Build history of the part. All positions in model axes, mm. A direction names the side the tool comes from. Give positions to 0.01 mm unless a question says otherwise; leave off trailing zeros. Order: outer loops, then holes, each group sorted by start corner. A loop starts at its lowest first (then second) coordinate and runs counter-clockwise, first axis right, second up. Notation, with made-up numbers: (87, -6) -> (106, -6) arc R34 ccw to (106, 29) -> close; hole circle Ø7 at (22, 76.25). An arc over 180 degrees is marked (long way). Use a Markdown table: item, result. Add a question column.
Autodesk Inventor part; units mm, degrees
ref_plane "YZ Plane" through (0, 0, 0) normal (1, 0, 0) x (0, 1, 0)
ref_plane "XZ Plane" through (0, 0, 0) normal (0, 1, 0) x (-1, 0, 0)
ref_plane "XY Plane" through (0, 0, 0) normal (0, 0, 1) x (1, 0, 0)
sketch "Sketch1" plane through (0, 0, 0) normal (0, 0, 1) x (1, 0, 0)
  line L0 (-750, 0) -> (750, 0) construction
  line L1 (750, 0) -> (750, -2700) construction
  line L2 (750, -2700) -> (-750, -2700) construction
  line L3 (-750, -2700) -> (-750, 0) construction
  line L4 (800, 50) -> (-800, 50) construction
  line L5 (-800, 50) -> (-800, -2750) construction
  line L6 (-800, -2750) -> (800, -2750) construction
  line L7 (800, -2750) -> (800, 50) construction
  line L8 (-850, 100) -> (850, 100) construction
  line L9 (850, 100) -> (850, -2800) construction
  line L10 (850, -2800) -> (-850, -2800) construction
  line L11 (-850, -2800) -> (-850, 100) construction
  arc A0 (750, 0) -> (745.2706, 0.6314) centre (0, -5600) ccw construction
  line L12 (-750, -2100) -> (750, -2100) construction
  line L13 (114.1118, -2698.3696) -> (687.3692, -2158.9354)
  arc A1 (750, -2100) -> (768.2917, -213.4901) centre (-10250, -1050) ccw construction
  line L14 (750, 0) -> (749.6018, -2.9735) construction
  arc A2 (750, -3.0268) -> (0, 47) centre (-0.2, -5603) ccw construction
  line L15 (750, 0) -> (747.0136, -0.2851) construction
  arc A3 (767.1641, -238.6409) -> (747.4657, -5.0326) centre (-10252.9895, -1050.2527) ccw construction
  arc A4 (750.4522, -4.7486) -> (745.2706, 0.6314) centre (744.4791, -5.3162) ccw construction
  arc A5 (747.4657, -5.0326) -> (744.8748, -2.3426) centre (744.4792, -5.3164) ccw construction
  line L16 (750, -2100) -> (752.9864, -2100.2851) construction
  arc A6 (752.9864, -2100.2851) -> (771.2831, -213.263) centre (-10246.9891, -1050.0292) ccw construction
  line L17 (750, -2100) -> (752.0559, -2102.1848) construction
  line L18 (752.0559, -2102.1848) -> (752.0559, -2102.1848) construction
  arc A7 (749.1768, -2100.7746) -> (750.1074, -2098.8746) centre (747.1209, -2098.5898) ccw construction
  line L19 (0, -2697) -> (110, -2697) construction
  line L20 (112.0559, -2696.1848) -> (685.3133, -2156.7506) construction
  arc A8 (110, -2700) -> (114.1118, -2698.3696) centre (110, -2694) ccw
  arc A9 (110, -2697) -> (112.0559, -2696.1848) centre (110, -2694) ccw construction
  line L21 (685.3133, -2156.7506) -> (687.3692, -2158.9354) construction
  line L22 (752.0559, -2102.1848) -> (671.2185, -2178.2526) construction
  line L23 (671.2185, -2178.2526) -> (669.1626, -2176.0678) construction
  arc A10 (747.4657, -5.0326) -> (747.0136, -0.2851) centre (-10252.9895, -1050.2527) ccw construction
  arc A11 (745.2706, 0.6314) -> (0, 50) centre (0, -5600) ccw construction
  arc A12 (750.4522, -4.7486) -> (750, 0) centre (-10250, -1050) ccw construction
  line L24 (770.156, -238.4205) -> (767.1641, -238.6409) construction
  line L25 (768.2917, -213.4901) -> (771.2831, -213.263) construction
  arc A13 (768.2917, -213.4901) -> (750.4522, -4.7486) centre (-10250, -1050) ccw construction
  line L26 (0, 100) -> (0, 50) construction
  line L27 (0, -2700) -> (0, -2697) construction
  line L28 (0, 47) -> (0, 0) construction
  line L29 (0, 50) -> (0, 47) construction
  arc A14 (752.0559, -2102.1848) -> (752.9864, -2100.2851) centre (749.9983, -2099.9992) ccw construction
  line L30 (0, -2700) -> (110, -2700)
  line L31 (687.3692, -2158.9354) -> (750, -2100) construction
  point P0 (0, -2750)
  dimension "d19" = 1500
  dimension "d20" = 2700
  dimension "d21" = 2100
  dimension "d22" = 6
  dimension "d23" = 3
  dimension "d24" = 3
  dimension "d25" = 6
  dimension "d26" = 3
  dimension "d27" = 239.271
  dimension "d28" = 50
  dimension "d29" = 50
  dimension "d30" = 3
  dimension "d31" = 25
  dimension "d32" = 110
  dimension "d33" = 25
  dimension "d34" = 111
contour flange "Contour Flange1" sketch "Sketch1" thickness 3 bend radius 3 width 1000 along (0, 0, 1) mid plane no both sides no wall seen from (55, -2700, 0) lies toward (0, 1, 0) curves L30 A8 L13
bend "Bend1"
corner "Corner1"
mirror "Mirror1" about plane through (0, 0, 0) normal (1, 0, 0)
equation "\"d19\" = Бак_ширина_общая"
equation "\"d20\" = Бак_высота_общая"
equation "\"d21\" = Бак_высота_до_конуса"
equation "\"d22\" = Thickness + BendRadius"
equation "\"d23\" = Thickness"
equation "\"d24\" = Thickness"
equation "\"d25\" = Thickness + BendRadius"
equation "\"d26\" = Thickness"
equation "\"d27\" = Бак_спина_длина_фланцев"
equation "\"d30\" = d40"
equation "\"d31\" = Бак_нахлест_фланца"
equation "\"d32\" = 0.5 * Бак_брюхо_ширина_полки"
equation "\"d33\" = Бак_нахлест_фланца"
equation "\"d34\" = Бак_борт_длина_фланца"
equation "\"d7\" = Thickness"
equation "\"d8\" = BendReliefWidth"
equation "\"d9\" = BendReliefDepth"
equation "\"d10\" = MinimumRemnant"
equation "\"d11\" = TransitionRadius"
equation "\"d13\" = BendRadius"
equation "\"d15\" = CornerReliefSize"
equation "\"d16\" = GapSize"
equation "\"d17\" = JacobiRadiusSize"
equation "\"BendRadius\" = Thickness"
equation "\"BendReliefWidth\" = Thickness"
equation "\"BendReliefDepth\" = 0.5 * Thickness"
equation "\"CornerReliefSize\" = 4 * Thickness"
equation "\"MinimumRemnant\" = 2 * Thickness"
equation "\"TransitionRadius\" = BendRadius"
equation "\"JacobiRadiusSize\" = BendRadius"
equation "\"GapSize\" = Thickness"
equation "\"d38\" = d40 + d44"
equation "\"d39\" = d40"
equation "\"d44\" = d40"
properties part number "МОО 041 sheet брюхо основной" material "Stainless Steel"
(1) Band-saw the part on B-B on y = -2456. Give the cut face in (x, z), plus the area to 3 significant figures.
(2) Pin check, flat tips, straight feed: pin 1 Ø3 at (x, z) = (183, 679) entering from -Y; pin 2 Ø2 at (y, z) = (-2587.5, 257.5) entering from -X; pin 3 Ø8 at (x, z) = (-426.5, 419.5) entering from +Y. Stop position of each tip, or through.
(3) Band-saw the part on C-C on x = -402. Give the cut face in (y, z), plus the area to 3 significant figures.
(4) Band-saw the part on A-A on z = 372. Give the cut face in (x, y), plus the area to 3 significant figures.
(5) Mould opens along X. For faces 1 (the face through (396.728, -2432.429, 493)), 2 (the face through (-2, -2697, 493)), 3 (the face through (-2, -2700, 493)) say: released by +X, released by -X, zero draft, split by the parting line, or undercut.
(6) Wall check: probe 1 along X at (y, z) = (-2270, 555.5); probe 2 along X at (y, z) = (-2423.5, 347.5); probe 3 along Y at (x, z) = (78.5, 500). Give the ranges that are in metal, low to high.
(7) Tool access for faces 4 (the face through (-404.75, -2424.88, 493)), 5 (the face through (-402.7, -2422.69, 493)): list every direction of +Z, -Z, +X, -X, +Y, -Y with a clear straight run to the whole face (end or side of a thin tool).
Response:
| question | item | result |
|---|---|---|
| 1 | outline | (-371.68, 0) -> (-367.3, 0) -> (-367.3, 1000) -> (-371.68, 1000) -> close; (367.3, 0) -> (371.68, 0) -> (371.68, 1000) -> (367.3, 1000) -> close |
| 1 | area | 8,760 mm² |
| 2 | pin 1 | stops at y = -2634.96 |
| 2 | pin 2 | stops at x = -233 |
| 2 | pin 3 | stops at y = -2396.53 |
| 3 | outline | (-2427.47, 0) -> (-2423.35, 0) -> (-2423.35, 1000) -> (-2427.47, 1000) -> close |
| 3 | area | 4,120 mm² |
| 4 | outline | (-687.37, -2158.94) -> (-114.11, -2698.37) arc R6 ccw to (-110, -2700) -> (110, -2700) arc R6 ccw to (114.11, -2698.37) -> (687.37, -2158.94) -> (685.31, -2156.75) -> (112.06, -2696.18) arc R3 cw to (110, -2697) -> (-110, -2697) arc R3 cw to (-112.06, -2696.18) -> (-685.31, -2156.75) -> close |
| 4 | area | 5,400 mm² |
| 5 | face 1 | released by +X |
| 5 | face 2 | undercut |
| 5 | face 3 | zero draft |
| 6 | probe 1 | x = -569.34 to -564.96, 564.96 to 569.34 |
| 6 | probe 2 | x = -406.22 to -401.84, 401.84 to 406.22 |
| 6 | probe 3 | y = -2700 to -2697 |
| 7 | face 4 | +Z, -Z, -X, -Y |
| 7 | face 5 | +Z, -Z, +Y |
